Part model, mm, in its own coordinate system. Round coordinates to 2 decimals unless told otherwise and drop trailing zeros. Write each loop counter-clockwise with the first axis right and the second up, starting at its lowest first coordinate (ties: lowest second). Pieces come first, ordered by that corner, then holes. Notation, with made-up numbers: M 87.25,-29 L 105.25,-29 A35 ccw 105.25,4 Z; hole C -13,13.5 d9. An arc over 180 degrees is marked long. Answer as a JSON object with one key per item and string values. Group by question number.
1. Drop flat-ended pins along their axis: pin 1 (1.5 mm diameter, centred on x = -72.5, y = 1.5, fed in from -Z); pin 2 (2 mm diameter, centred on y = 2.5, z = -108, fed in from -X). Give the stop position or say it passes through.
2. Drill centre lines: line 1 (Z direction, x = 168.5, y = 3); line 2 (Z direction, x = 4, y = 3.55); line 3 (X direction, y = 0.25, z = -60.5). Where is each one in solid material? Low to high. Write a range as from..to.
3. Band-saw the part on B-B, the plane x = -72. Write the cut outline in (y, z), plus the area to 3 significant figures.
4. Band-saw the part on C-C, the plane z = -31. Write the cut outline in (x, y), plus the area to 3 significant figures.
5. Band-saw the part on A-A, the plane y = 2.55. Count the separate pieces of the cut face and the enclosed holes in it, plus the area to 3 significant figures.
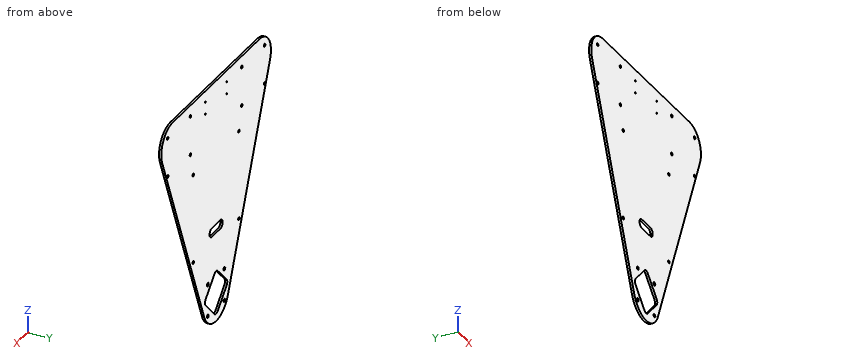
from build123d import *

# Parameters (mm, degrees)
SKETCH_2_R      = 3.1
SKETCH_2_R_2    = 2.65
SKETCH_2_R_3    = 1.35
SKETCH_2_R_4    = 2.6
EXTRUDE_2_DEPTH = 4


with BuildPart() as part:
    # 草图2 → 凸台-拉伸2 (new body)
    with BuildSketch(Plane(origin=(0, 0, 0), x_dir=(1, 0, 0), z_dir=(0, 1, 0))):
        with BuildLine():
            Line((-41.574578963, 199.630087618), (-189.22298515, -156.824697061))
            ThreePointArc((-189.22298515, -156.824697061), (-185.526588341, -194.354843677), (-152.267803849, -212.132034356))
            Line((-152.267803849, -212.132034356), (152.267803849, -212.132034356))
            ThreePointArc((152.267803849, -212.132034356), (185.526588341, -194.354843677), (189.22298515, -156.824697061))
            Line((189.22298515, -156.824697061), (41.574578963, 199.630087618))
            ThreePointArc((41.574578963, 199.630087618), (0, 227.409333161), (-41.574578963, 199.630087618))
        make_face()
        with Locations(Location((28.991378029, 203.991378029, 0), (0, 0, 270))):
            Circle(SKETCH_2_R, mode=Mode.SUBTRACT)
        with Locations(Location((-28.991378029, 203.991378029, 0), (0, 0, 90))):
            Circle(SKETCH_2_R, mode=Mode.SUBTRACT)
        with Locations(Location((28.991378029, 146.008621971, 0), (0, 0, 90))):
            Circle(SKETCH_2_R, mode=Mode.SUBTRACT)
        with Locations(Location((-28.991378029, 146.008621971, 0), (0, 0, 270))):
            Circle(SKETCH_2_R, mode=Mode.SUBTRACT)
        with Locations(Location((-170, -122.132034356, 0), (0, 0, 270))):
            Circle(SKETCH_2_R_2, mode=Mode.SUBTRACT)
        with Locations(Location((-90, -122.132034356, 0), (0, 0, 270))):
            Circle(SKETCH_2_R_2, mode=Mode.SUBTRACT)
        with Locations(Location((-90, -192.132034356, 0), (0, 0, 270))):
            Circle(SKETCH_2_R_2, mode=Mode.SUBTRACT)
        with Locations(Location((-170, -192.132034356, 0), (0, 0, 270))):
            Circle(SKETCH_2_R_2, mode=Mode.SUBTRACT)
        with Locations(Location((90, -192.132034356, 0), (0, 0, 90))):
            Circle(SKETCH_2_R_2, mode=Mode.SUBTRACT)
        with Locations(Location((170, -192.132034356, 0), (0, 0, 90))):
            Circle(SKETCH_2_R_2, mode=Mode.SUBTRACT)
        with Locations(Location((90, -122.132034356, 0), (0, 0, 90))):
            Circle(SKETCH_2_R_2, mode=Mode.SUBTRACT)
        with Locations(Location((170, -122.132034356, 0), (0, 0, 90))):
            Circle(SKETCH_2_R_2, mode=Mode.SUBTRACT)
        with Locations(Location((37.5, -170.132034356, 0), (0, 0, 270))):
            Circle(SKETCH_2_R_3, mode=Mode.SUBTRACT)
        with Locations(Location((-37.5, -170.132034356, 0), (0, 0, 270))):
            Circle(SKETCH_2_R_3, mode=Mode.SUBTRACT)
        with Locations(Location((-37.5, -192.132034356, 0), (0, 0, 270))):
            Circle(SKETCH_2_R_3, mode=Mode.SUBTRACT)
        with Locations(Location((37.5, -192.132034356, 0), (0, 0, 270))):
            Circle(SKETCH_2_R_3, mode=Mode.SUBTRACT)
        with Locations(Location((-80, 80, 0), (0, 0, 270))):
            Circle(SKETCH_2_R_4, mode=Mode.SUBTRACT)
        with Locations(Location((80, 80, 0), (0, 0, 270))):
            Circle(SKETCH_2_R_4, mode=Mode.SUBTRACT)
        with Locations(Location((80, -80, 0), (0, 0, 270))):
            Circle(SKETCH_2_R_4, mode=Mode.SUBTRACT)
        with Locations(Location((-80, -80, 0), (0, 0, 270))):
            Circle(SKETCH_2_R_4, mode=Mode.SUBTRACT)
        with BuildLine():
            Line((-36.769552622, 180.656854249), (-5.656854249, 211.769552622))
            ThreePointArc((-5.656854249, 211.769552622), (0, 214.112698372), (5.656854249, 211.769552622))
            Line((5.656854249, 211.769552622), (36.769552622, 180.656854249))
            ThreePointArc((36.769552622, 180.656854249), (39.112698372, 175), (36.769552622, 169.343145751))
            Line((36.769552622, 169.343145751), (5.656854249, 138.230447378))
            ThreePointArc((5.656854249, 138.230447378), (0, 135.887301628), (-5.656854249, 138.230447378))
            Line((-5.656854249, 138.230447378), (-36.769552622, 169.343145751))
            ThreePointArc((-36.769552622, 169.343145751), (-39.112698372, 175), (-36.769552622, 180.656854249))
        make_face(mode=Mode.SUBTRACT)
        with BuildLine():
            Line((-15, 65.867965644), (15, 65.867965644))
            ThreePointArc((15, 65.867965644), (23, 57.867965644), (15, 49.867965644))
            Line((15, 49.867965644), (-15, 49.867965644))
            ThreePointArc((-15, 49.867965644), (-23, 57.867965644), (-15, 65.867965644))
        make_face(mode=Mode.SUBTRACT)
    extrude(amount=EXTRUDE_2_DEPTH)


solid = part.part
Worked answers:
{
 "1": {"pin 1": "stops at z = -126.78", "pin 2": "stops at x = -79.94"},
 "2": {"line 1": "z = 106.79..119.95, 124.32..189.95, 194.32..208.69", "line 2": "z = -227.23..-213.04, -136.96..-65.87, -49.87..212.13", "line 3": "x = -99.2..-22.55, 22.55..99.2"},
 "3": {"outline": "M 0,-126.18 L 4,-126.18 L 4,212.13 L 0,212.13 Z", "area": "1,350 mm^2"},
 "4": {"outline": "M -111.42,0 L 111.42,0 L 111.42,4 L -111.42,4 Z", "area": "891 mm^2"},
 "5": {"separate pieces": "1", "enclosed holes": "22", "area": "99,900 mm^2"}
}
